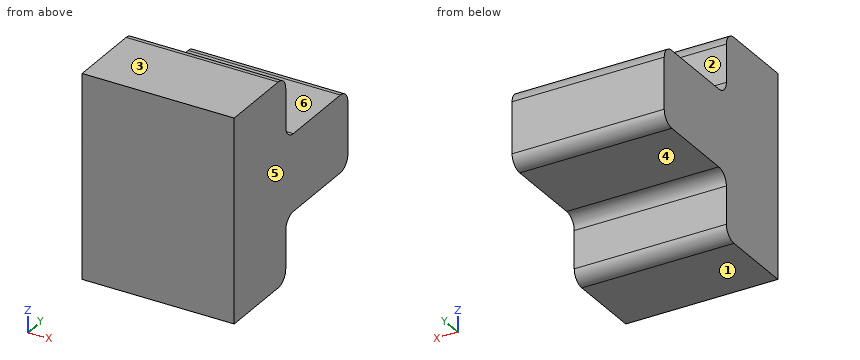
```python
from build123d import *

# Parameters (mm, degrees)
BOSS_EXTRUDE1_DEPTH  = 12
FILLET1_R            = 1
FILLET1_OF_MIRROR2_R = 1


with BuildPart() as part:
    # Sketch1 → Boss-Extrude1 (new body)
    with BuildSketch(Plane(origin=(0, 0, 0), x_dir=(0, 0, -1), z_dir=(1, 0, 0))):
        Polygon((0, 6.800479655), (0, 0), (8, 0), (8, 15), (4.975646797, 15), (4.975646797, 6.800479655), align=None)
    boss_extrude1 = extrude(amount=BOSS_EXTRUDE1_DEPTH)

    # Fillet1
    fillet1_edges = [part.edges().sort_by_distance(p)[0] for p in [
        (6, 6.800479655, 0),
        (6, 6.800479655, -4.975646797),
        (6, 15, -4.975646797),
    ]]
    fillet(fillet1_edges, radius=FILLET1_R)

    # Mirror2: Boss-Extrude1 across plane
    add(boss_extrude1.mirror(Plane(origin=(12, 0, -8), x_dir=(1, 0, 0), z_dir=(0, 0, 1))))

    # Fillet1 of Mirror2
    fillet1_of_mirror2_edges = [part.edges().sort_by_distance(p)[0] for p in [
        (6, 6.800479655, -16),
        (6, 6.800479655, -11.024353203),
        (6, 15, -11.024353203),
    ]]
    fillet(fillet1_of_mirror2_edges, radius=FILLET1_OF_MIRROR2_R)


solid = part.part
```
The listing builds one solid part. Answer for the finished solid, in the listing's coordinates (mm). Face numbers are marked on the shaded views. A direction names the side the tool comes from. Coordinates: 2 decimals unless noted, no trailing zeros. Loops run counter-clockwise (first coordinate to the right, second up) from the corner with the lowest first, then second, coordinate; pieces in that order, holes last. Notation, with made-up numbers: (-10, -21.5) - (-2, -21.5) arc R21 ccw to (-2, 0.5) - close; hole circle Ø9 at (70, 25). An arc over 180 degrees is marked (long way). Use a Markdown table: item, result. Add a question column.
1) Given pin 1 (1.5 mm diameter, centred on x = 6, z = -13, fed in from +Y); pin 2 (1.5 mm diameter, centred on x = 1.5, y = 8.5, fed in from +Z); pin 3 (1.5 mm diameter, centred on x = 2.5, y = 7, fed in from -Z), each flat-ended and moving along its own axis, determine where each tip first touches the part or whether it passes through.
2) Find the intervals of material crossed by line 1 (Z direction, x = 2.75, y = 11.5); line 2 (Y direction, x = 6, z = -15); line 3 (Y direction, x = 10.25, z = -5.75), in increasing order.
3) The part is cut by section B-B, the plane z = -1.25. Give the vertices of the cut face in (x, y), and give its area (3 significant figures).
4) The part is cut by section C-C, the plane y = 11. Give the vertices of the cut face in (x, z).
5) For the marked faces 4, 5 and 6, determine the directions among +Z, -Z, +X, -X, +Y, -Y from which every point of the face is accessible in a straight line to the end or side of a thin tool.
6) The part is cut by section A-A, the plane x = 5. Give the vertices of the cut face in (y, z).
7) The mould has two halves that part along Z. Classify the marked faces 1, 2 and 3: released by +Z, released by -Z, zero draft, split by the parting line, or undercut.
Here are the results:
| question | item | result |
|---|---|---|
| 1 | pin 1 | stops at y = 6.8 |
| 1 | pin 2 | stops at z = -4.97 |
| 1 | pin 3 | stops at z = -15.89 |
| 2 | line 1 | z = -11.02 to -4.98 |
| 2 | line 2 | y = 0 to 6.8 |
| 2 | line 3 | y = 0 to 14.97 |
| 3 | outline | (0, 0) - (12, 0) - (12, 6.8) - (0, 6.8) - close |
| 3 | area | 81.6 mm^2 |
| 4 | outline | (0, -11.02) - (12, -11.02) - (12, -4.98) - (0, -4.98) - close |
| 5 | face 4 | -Z, +X, -X, +Y |
| 5 | face 5 | +Z, -Z, +X, +Y, -Y |
| 5 | face 6 | +Z, +X, -X, +Y |
| 6 | outline | (0, -16) - (5.8, -16) arc R1 ccw to (6.8, -15) - (6.8, -12.02) arc R1 cw to (7.8, -11.02) - (14, -11.02) arc R1 ccw to (15, -10.02) - (15, -5.98) arc R1 ccw to (14, -4.98) - (7.8, -4.98) arc R1 cw to (6.8, -3.98) - (6.8, -1) arc R1 ccw to (5.8, 0) - (0, 0) - close |
| 7 | face 1 | released by -Z |
| 7 | face 2 | zero draft |
| 7 | face 3 | released by +Z |
